Input: part model. Units: mm. Frame: model coordinates. A direction names the side the tool comes from. Give positions to 0.01 mm unless a question says otherwise; leave off trailing zeros. Loops run counter-clockwise (first coordinate to the right, second up) from the corner with the lowest first, then second, coordinate; pieces in that order, holes last. Notation, with made-up numbers: (-19, 78) -> (4, 78) arc R36 ccw to (4, 116) -> close; hole circle Ø10 at (-32.5, -15). An arc over 180 degrees is marked (long way). Use CSV: the item, a comma, the result in double quotes.
```python
from build123d import *

# Parameters (mm, degrees)
BOSS_EXTRUDE1_DEPTH      = 137.5
BOSS_EXTRUDE1_DEPTH_BACK = 137.5


with BuildPart() as part:
    # Sketch1 → Boss-Extrude1 (new, two sides: drawn at the far end of the back side and taken through both)
    with BuildSketch(Plane(origin=(0, 0, 0), x_dir=(0, 0, -1), z_dir=(1, 0, 0)).offset(-BOSS_EXTRUDE1_DEPTH_BACK)):
        with BuildLine():
            Line((0, -10), (0, -0.5))
            ThreePointArc((0, -0.5), (0.146446609, -0.146446609), (0.5, 0))
            Line((0.5, 0), (10, 0))
            Line((10, 0), (10, -0.5))
            Line((10, -0.5), (1, -0.5))
            ThreePointArc((1, -0.5), (0.646446609, -0.646446609), (0.5, -1))
            Line((0.5, -1), (0.5, -10))
            Line((0.5, -10), (0, -10))
        make_face()
    extrude(amount=BOSS_EXTRUDE1_DEPTH + BOSS_EXTRUDE1_DEPTH_BACK)


solid = part.part
```
1) Section query B-B (y = -5). Return loops of the section in (x, z), then the cut area to 4 significant figures.
From the geometry:
outline,"(-137.5, -0.5) -> (137.5, -0.5) -> (137.5, 0) -> (-137.5, 0) -> close"
area,"137.5 mm^2"
2) Section query A-A (x = 98.5). Return loops of the section in (y, z).
From the geometry:
outline,"(-10, -0.5) -> (-1, -0.5) arc R0.5 cw to (-0.5, -1) -> (-0.5, -10) -> (0, -10) -> (0, -0.5) arc R0.5 ccw to (-0.5, 0) -> (-10, 0) -> close"
3) Reachability of faces 1 (the flat face through (-2, 0, -5)), 2 (the flat face through (-2, -0.5, -6)) from +Z, -Z, +X, -X, +Y, -Y: full face, straight path, thin tool, end or side. Return the list, or none.
From the geometry:
face 1,"+Z, -Z, +X, -X, +Y"
face 2,"-Z, +X, -X, -Y"
4) Ray query, line 1 (Z direction, x = -28, y = -3.5). Return the intervals inside material, ascending.
From the geometry:
line 1,"z = -0.5 to 0"
5) Contact query for flat-ended pins moving along their axis: pin 1 (2 mm diameter, centred on x = -32.5, y = -3, fed in from -Z); pin 2 (1 mm diameter, centred on x = 56.5, z = -2, fed in from -Y). Output: stop coordinate, or through.
From the geometry:
pin 1,"stops at z = -0.5"
pin 2,"stops at y = -0.5"
